Could you check a few things on this model? Use its own coordinates, in mm. A direction names the side the tool comes from. Coordinates: 2 decimals unless noted, no trailing zeros. Order: outer loops, then holes, each group sorted by start corner. A loop starts at its lowest first (then second) coordinate and runs counter-clockwise, first axis right, second up.
Autodesk Inventor part; units mm, degrees
ref_plane "YZ Plane" through (0, 0, 0) normal (1, 0, 0) x (0, 1, 0)
ref_plane "XZ Plane" through (0, 0, 0) normal (0, 1, 0) x (-1, 0, 0)
ref_plane "XY Plane" through (0, 0, 0) normal (0, 0, 1) x (1, 0, 0)
sketch "Sketch1" plane through (0, 0, 0) normal (0, 0, 1) x (1, 0, 0)
  arc A0 (6.3455, 7.6592) -> (2.9969, 4.161) centre (5.1207, 5.4798) ccw
  arc A1 (28.9309, -45.2636) -> (10.279, 5.1864) centre (-16.779, -33.4901) ccw
  arc A2 (8.9309, -45.2636) -> (6.4804, -0.2246) centre (-28.4708, -24.7125) ccw
  line L0 (8.9309, -45.2636) -> (28.9309, -45.2636)
  line L1 (22.9916, -36.6135) -> (18.8703, -36.6135)
  line L2 (22.9916, -39.6135) -> (18.8703, -39.6135)
  line L3 (20.9309, -34.0784) -> (20.9309, -41.4431) construction
  line L4 (22.8639, -38.1135) -> (15.5009, -38.1135) construction
  arc A3 (18.8703, -36.6135) -> (18.8703, -39.6135) centre (20.9309, -38.1135) ccw
  arc A4 (22.9916, -39.6135) -> (22.9916, -36.6135) centre (20.9309, -38.1135) ccw
  line L5 (18.6071, -36.0635) -> (23.2547, -36.0635)
  arc A5 (23.2547, -40.1635) -> (23.2547, -36.0635) centre (20.9309, -38.1135) ccw
  line L6 (23.2547, -40.1635) -> (18.6071, -40.1635)
  arc A6 (18.6071, -36.0635) -> (18.6071, -40.1635) centre (20.9309, -38.1135) ccw
  arc A7 (2.9969, 4.161) -> (6.4804, -0.2246) centre (4.7985, 2.0157) ccw
  arc A8 (10.279, 5.1864) -> (5.805, 7.8843) centre (7.5999, 5.8022) ccw
  point P0 (0, 0)
  dimension "d25" = 2.5
  dimension "d32" = 20
  dimension "d40" = 1.5
  dimension "d41" = 1.5
  dimension "d42" = 8
  dimension "d43" = 7.1502
  dimension "d44" = 0.55
extrude "Extrusion1" add sketch "Sketch1" along normal blind 5 contours A8 A1 L0 A2 A7 A0
sketch "Sketch3" plane through (0, 0, 0) normal (0, 0, -1) x (-1, 0, 0)
  line L0 (-18.6071, -36.0635) -> (-23.2547, -36.0635)
  arc A0 (-23.2547, -36.0635) -> (-23.2547, -40.1635) centre (-20.9309, -38.1135) ccw
  line L1 (-23.2547, -40.1635) -> (-18.6071, -40.1635)
  arc A1 (-18.6071, -40.1635) -> (-18.6071, -36.0635) centre (-20.9309, -38.1135) ccw
  line L2 (-23.8543, -34.5635) -> (-18.0075, -34.5635)
  arc A2 (-18.0075, -41.6635) -> (-18.0075, -34.5635) centre (-20.9309, -38.1135) ccw
  line L3 (-18.0075, -41.6635) -> (-23.8543, -41.6635)
  arc A3 (-23.8543, -34.5635) -> (-23.8543, -41.6635) centre (-20.9309, -38.1135) ccw
  point P0 (0, 0)
  dimension "d45" = 1.5
extrude "Extrusion3" add sketch "Sketch3" along normal blind 5
fillet "Fillet2" radius 7 2 edges at (8.9309, -45.2636, 2.5) (28.9309, -45.2636, 2.5)
properties part number "mavac_ruka I guesss"
Item 1: Suppose I cut it at A-A (x = 20.25). List the corners of the cut face in (y, z) for me, and give its area (3 significant figures).
Item 2: For pin 1 Ø4 at (x, z) = (22.5, -3.5) entering from +Y; pin 2 Ø12 at (x, y) = (23, -23.5) entering from -Z; pin 3 Ø5 at (x, z) = (21.5, -1.5) entering from +Y, each with a flat end and sliding along its axis, tell me the tip position at first contact or that it passes through.
Item 3: Suppose I cut it at C-C (y = -14). List the corners of the cut face in (x, z) for me, and give its area (3 significant figures).
Item 4: Suppose I cut it at D-D (x = 9). List the corners of the cut face in (y, z) for me.
Item 5: Thinking about a two-plate mould opening in X: for faces 4 (the face through (21, -45.264, 2)), 5 (the face through (21, -36.064, 0)), 6 (the face through (26.16, -13.89, 2.46)), 7 (the face through (13.68, -42.41, 2.54)), which applies, +X half, -X half, draft (parallel to the pull), parting line (faces both ways), or undercut?
Item 6: I need wall thicknesses on line 1 (Z direction, x = 18, y = -4); line 2 (X direction, y = -38, z = -3.25); line 3 (Y direction, x = 22.5, z = 3.5). Which ranges of each line are inside material? Lowest first, please.
Item 7: Which directions (+Z, -Z, +X, -X, +Y, -Y) give clear straight access to the entire face, cutting with the end or side of a thin tool? Please do faces 1 (the face through (25.53, -38.17, -2.46)), 2 (the face through (21, -34.564, -2)), 3 (the face through (21, -40.164, 0)).
Item 8: Suppose I cut it at B-B (z = -2.75). List the corners of the cut face in (x, y) for me, and give its area (3 significant figures).
Geometry results:
1. outline: (-45.26, 0) - (-41.66, 0) - (-41.66, -5) - (-40.16, -5) - (-40.16, 5) - (-45.26, 5) - close; (-36.06, -5) - (-34.56, -5) - (-34.56, 0) - (-4.22, 0) - (-4.22, 5) - (-36.06, 5) - close
1. area: 200 mm2
2. pin 1: stops at y = -34.56
2. pin 2: stops at z = 0
2. pin 3: stops at y = -3.29
3. outline: (12.84, 0) - (26.21, 0) - (26.21, 5) - (12.84, 5) - close
3. area: 66.9 mm2
4. outline: (-4.29, 0) - (8.17, 0) - (8.17, 5) - (-4.29, 5) - close
5. face 4: draft
5. face 5: undercut
5. face 6: +X half
5. face 7: -X half
6. line 1: z = 0 to 5
6. line 2: x = 16.33 to 17.83, 24.03 to 25.53
6. line 3: y = -45.26 to -40.16, -36.06 to -7.31
7. face 1: -Z, +X
7. face 2: -Z, +X, -X, +Y
7. face 3: +Z, -Z
8. outline: (18.01, -41.66) - (23.85, -41.66) arc R4.6 ccw to (23.85, -34.56) - (18.01, -34.56) arc R4.6 ccw to start; hole (18.61, -40.16) - (23.25, -40.16) arc R3.1 ccw to (23.25, -36.06) - (18.61, -36.06) arc R3.1 ccw to start
8. area: 34.6 mm2
